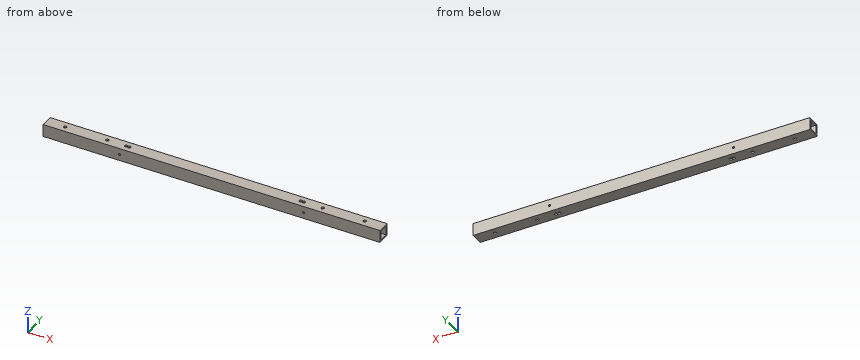
Autodesk Inventor part; units mm, degrees
ref_plane "YZ Plane" through (0, 0, 0) normal (1, 0, 0) x (0, 1, 0)
ref_plane "XZ Plane" through (0, 0, 0) normal (0, 1, 0) x (-1, 0, 0)
ref_plane "XY Plane" through (0, 0, 0) normal (0, 0, 1) x (1, 0, 0)
sketch "Sketch1" plane through (0, 0, 0) normal (1, 0, 0) x (0, 1, 0)
  line L0 (0, 0) -> (25.4, 0)
  line L1 (25.4, 0) -> (25.4, -25.4)
  line L2 (25.4, -25.4) -> (0, -25.4)
  line L3 (0, -25.4) -> (0, 0)
  line L4 (3.175, -3.175) -> (22.225, -3.175)
  line L5 (22.225, -3.175) -> (22.225, -22.225)
  line L6 (22.225, -22.225) -> (3.175, -22.225)
  line L7 (3.175, -22.225) -> (3.175, -3.175)
  dimension "d0" = 25.4
  dimension "d1" = 25.4
  dimension "d2" = 19.05
  dimension "d3" = 19.05
  dimension "d4" = 3.175
  dimension "d5" = 3.175
extrude "Extrusion1" add sketch "Sketch1" along normal blind 685.8
sketch "Sketch3" plane through (0, 0, -25.4) normal (0, 0, -1) x (-1, 0, 0)
  line L0 (0, 25.4) -> (0, 0)
  line L1 (-685.8, 0) -> (-685.8, 25.4)
  line L2 (0, 0) -> (-685.8, 0)
  point P0 (-647.7, 12.7)
  point P1 (-561.975, 12.7)
  point P2 (-523.875, 12.7)
  point P3 (-161.925, 12.7)
  point P4 (-123.825, 12.7)
  point P5 (-38.1, 12.7)
  dimension "d23" = 38.1
  dimension "d24" = 12.7
  dimension "d25" = 12.7
  dimension "d26" = 12.7
  dimension "d27" = 123.825
  dimension "d28" = 161.925
  dimension "d29" = 12.7
  dimension "d30" = 12.7
  dimension "d31" = 12.7
  dimension "d32" = 38.1
  dimension "d33" = 123.825
  dimension "d34" = 161.925
hole "Hole2" at (647.7, 12.7, -25.4) at (561.975, 12.7, -25.4) at (523.875, 12.7, -25.4) at (161.925, 12.7, -25.4) at (123.825, 12.7, -25.4) at (38.1, 12.7, -25.4) direction (0, 0, 1) diameter 6.35 end through all
sketch "Sketch6" plane through (0, 0, -25.4) normal (0, 0, -1) x (-1, 0, 0)
  circle A0 centre (-523.875, 12.7) radius 3.175
  circle A1 centre (-161.925, 12.7) radius 3.175
  line L0 (0, 0) -> (-685.8, 0)
  circle A2 centre (-517.525, 12.7) radius 3.175
  circle A3 centre (-168.275, 12.7) radius 3.175
  dimension "d66" = 6.35
  dimension "d67" = 6.35
  dimension "d68" = 12.7
  dimension "d69" = 6.35
  dimension "d70" = 6.35
  dimension "d71" = 12.7
extrude "Extrusion2" cut sketch "Sketch6" against normal blind 25.4 contours A2 | A3
sketch "Sketch7" plane through (0, 25.4, 0) normal (0, 1, 0) x (1, 0, 0)
  line L0 (685.8, 25.4) -> (685.8, 0)
  line L1 (0, 25.4) -> (685.8, 25.4)
  point P0 (155.575, 12.7)
  point P1 (530.225, 12.7)
  dimension "d74" = 12.7
  dimension "d75" = 12.7
  dimension "d76" = 530.225
  dimension "d77" = 155.575
hole "Hole5" at (155.575, 25.4, -12.7) at (530.225, 25.4, -12.7) direction (0, -1, 0) diameter 4.7625 depth 25.4 tip angle 118
properties part number "1x1 horizontal lower" material "Aluminum 6061"
The listing builds one solid part. Answer for the finished solid, in the listing's coordinates (mm). Round coordinates to 2 decimals unless told otherwise and drop trailing zeros. Loops run counter-clockwise (first coordinate to the right, second up) from the corner with the lowest first, then second, coordinate; pieces in that order, holes last. Notation, with made-up numbers: (53, -11.5) -> (83, -11.5) arc R7 ccw to (83, 0.5) -> close; hole circle Ø9 at (6.25, 76.5). An arc over 180 degrees is marked (long way). Use one line per item in the form item = value.
1. The part is cut by section A-A on x = 365. Determine the outline of the cut face in (y, z) (3 decimals), and give its area (3 significant figures).
Answer key:
outline = (0, -25.4) -> (25.4, -25.4) -> (25.4, 0) -> (0, 0) -> close; hole (3.175, -22.225) -> (22.225, -22.225) -> (22.225, -3.175) -> (3.175, -3.175) -> close
area = 282 mm²
2. Flat-ended cylindrical pins translate along their axes: pin 1 Ø8.5 at (x, y) = (647.7, 12.7) entering from +Z; pin 2 Ø5 at (x, y) = (523.875, 12.7) entering from -Z. Find the tip coordinate at first contact, or state that the pin passes through.
Answer key:
pin_1 = 0
pin_2 = through
3. Find the intervals of material crossed by probe 1 along Z at (x, y) = (428.5, 14) (3 decimals); probe 2 along Y at (x, z) = (537, -5.75) (3 decimals); probe 3 along Y at (x, z) = (38.1, -2.3) (3 decimals), in increasing order. Write a range as [from, to].
Answer key:
probe_1 = [-25.4, -22.225], [-3.175, 0]
probe_2 = [0, 3.175], [22.225, 25.4]
probe_3 = [0, 9.525], [15.875, 25.4]
